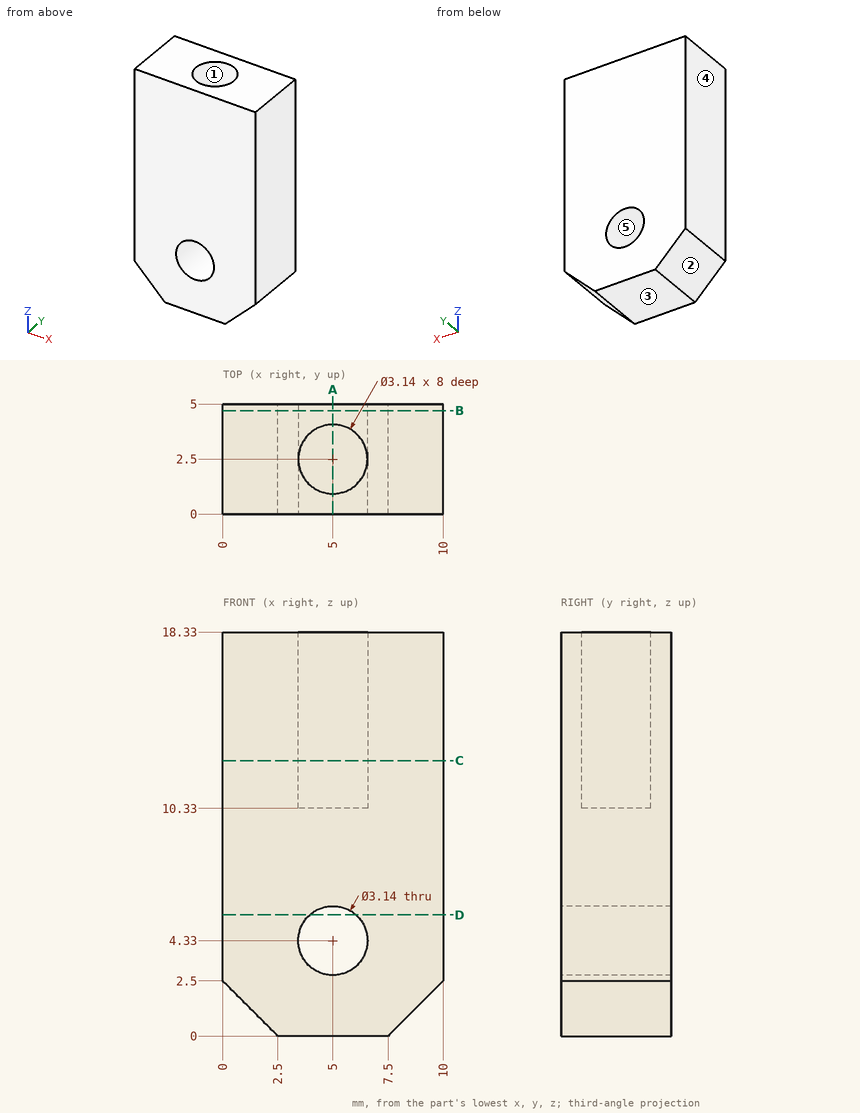
The drawing under review shows one solid part. Ordinate dimensions are in mm from its lowest x, y, z. A direction names the side the tool comes from. Coordinates: 2 decimals unless noted, no trailing zeros. Order: outer loops, then holes, each group sorted by start corner. A loop starts at its lowest first (then second) coordinate and runs counter-clockwise, first axis right, second up. Notation, with made-up numbers: (60, 34.5) -> (108, 34.5) arc R28 cw to (108, 71.5) -> close; hole circle Ø2 at (76.25, 77). An arc over 180 degrees is marked (long way). Answer in a Markdown table with one row per item. Add a question column.
Item 1: We need section B-B on y = 4.7. Write out the cut boundary in (x, z).
Item 2: We need section C-C on z = 12.5. Write out the cut boundary in (x, y).
Item 3: Machinability: for the marked faces 1 and 2, which of the approach directions +Z, -Z, +X, -X, +Y, -Y give a long, thin tool a straight path to every point of the face, cutting with its end or side? Answer none if there is none.
Item 4: We need section A-A on x = 5. Write out the cut boundary in (y, z), plus the area to 3 significant figures.
Item 5: We need section D-D on z = 5.5. Write out the cut boundary in (x, y), plus the area to 3 significant figures.
Item 6: Mouldability with a two-part tool opening along X and no side actions: class the marked faces 3, 4 and 5 as +X half, -X half, draft (parallel to the pull), parting line (faces both ways), or undercut.
Item 7: To check wall thickness, follow probe 1 along X at (y, z) = (3.4, 14.5); probe 2 along Z at (x, y) = (5, 3.5); probe 3 along Y at (x, z) = (5, 16.25). State the ranges of each line that lie inside material, in increasing order.
Item 8: Clearance check with flat-ended pins moving along their axes: pin 1 (2 mm diameter, centred on x = 8.5, z = 3, fed in from -Y); pin 2 (1.6 mm diameter, centred on x = 5.5, y = 3, fed in from +Z). State where each tip first meets the part, or that it passes through.
Final values:
| question | item | result |
|---|---|---|
| 1 | outline | (0, 2.5) -> (2.5, 0) -> (7.5, 0) -> (10, 2.5) -> (10, 18.33) -> (0, 18.33) -> close; hole circle Ø3.14 at (5, 4.33) |
| 2 | outline | (0, 0) -> (10, 0) -> (10, 5) -> (0, 5) -> close; hole circle Ø3.14 at (5, 2.5) |
| 3 | face 1 | +Z |
| 3 | face 2 | -Z, -X, +Y, -Y |
| 4 | outline | (0, 0) -> (5, 0) -> (5, 2.76) -> (0, 2.76) -> close; (0, 5.9) -> (5, 5.9) -> (5, 18.33) -> (4.07, 18.33) -> (4.07, 10.33) -> (0.93, 10.33) -> (0.93, 18.33) -> (0, 18.33) -> close |
| 4 | area | 50.8 mm2 |
| 5 | outline | (0, 0) -> (3.95, 0) -> (3.95, 5) -> (0, 5) -> close; (6.05, 0) -> (10, 0) -> (10, 5) -> (6.05, 5) -> close |
| 5 | area | 39.5 mm2 |
| 6 | face 3 | draft |
| 6 | face 4 | -X half |
| 6 | face 5 | undercut |
| 7 | probe 1 | x = 0 to 3.71, 6.29 to 10 |
| 7 | probe 2 | z = 0 to 2.76, 5.9 to 10.33 |
| 7 | probe 3 | y = 0 to 0.93, 4.07 to 5 |
| 8 | pin 1 | stops at y = 0 |
| 8 | pin 2 | stops at z = 10.33 |
